Input: dimensioned drawing with shaded views. Units: mm. Origin: part minimum x, y, z. Give positions to 0.01 mm unless a question says otherwise; leave off trailing zeros. Write each loop counter-clockwise with the first axis right and the second up, starting at its lowest first coordinate (ties: lowest second). Pieces come first, ordered by that corner, then holes. Notation, with made-up numbers: (20, 56.5) -> (59, 56.5) arc R19 cw to (59, 74.5) -> close; hole circle Ø1 at (66, 28.5). An arc over 180 degrees is marked (long way). Return JSON: item names as keys, results as strings. Group by question number.
Item 1: Line query: line 1 (X direction, y = 18.5, z = 11.25); line 2 (X direction, y = 1.5, z = 1.75); line 3 (X direction, y = 7, z = 13.5). Output: solid intervals per line, ascending. Write a range as [from, to].
Item 2: Pin query (flat end, axial travel): P1, Ø6, axis at y = 8.5, z = 21, coming from the +X side; P2, Ø1.5, axis at x = 252, z = 7.5, coming from the +Y side; P3, Ø4, axis at y = 8, z = 7.5, coming from the -X side; P4, Ø10, axis at x = 12.7, z = 12.7, coming from the -Y side. Return the tip coordinate at first contact, or that it passes through.
Item 3: Section B-B, the plane y = 9. Return loops of the section in (x, z) (3 decimals).
Item 4: Section C-C, the plane x = 792. Return loops of the section in (y, z) (3 decimals).
Item 5: Section A-A, the plane z = 12.7. Return loops of the section in (x, y) (3 decimals).
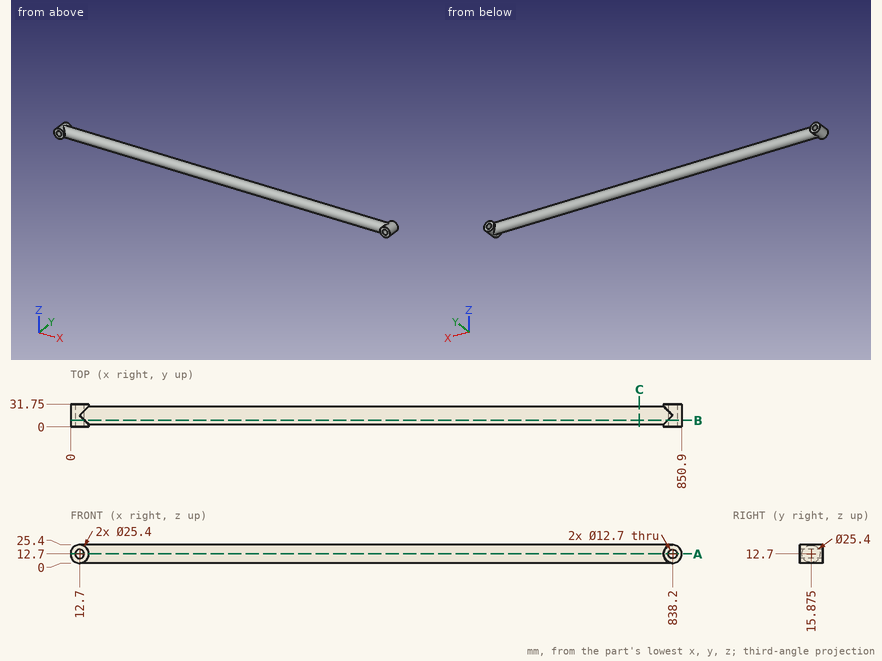
Answer below:
{
 "1": {"line 1": "x = [0.08, 6.52], [18.88, 832.02], [844.38, 850.82]", "line 2": "x = [6.27, 19.13], [831.77, 844.63]", "line 3": "x = [0.03, 6.4], [19, 831.9], [844.5, 850.87]"},
 "2": {"P1": "stops at x = 849.74", "P2": "stops at y = 27.77", "P3": "stops at x = 0.41", "P4": "passes through"},
 "3": {"outline": "(19.575, 2.022) -> (831.325, 2.022) arc R12.7 ccw (long way) to (831.325, 23.378) -> (19.575, 23.378) arc R12.7 ccw (long way) to start; hole circle Ø12.7 at (12.7, 12.7); hole circle Ø12.7 at (838.2, 12.7)"},
 "4": {"outline": "circle Ø25.4 at (15.875, 12.7)"},
 "5": {"outline": "(0, 0) -> (6.35, 0) -> (6.35, 31.75) -> (0, 31.75) -> close; (19.05, 0) -> (25.4, 0) -> (25.4, 3.175) -> (825.5, 3.175) -> (825.5, 0) -> (831.85, 0) -> (831.85, 31.75) -> (825.5, 31.75) -> (825.5, 28.575) -> (25.4, 28.575) -> (25.4, 31.75) -> (19.05, 31.75) -> close; (844.55, 0) -> (850.9, 0) -> (850.9, 31.75) -> (844.55, 31.75) -> close"}
}
